Study the drawing (mm; zero at the part's minimum x, y, z) and answer. Give positions to 0.01 mm unless a question says otherwise; leave off trailing zeros. Write each loop counter-clockwise with the first axis right and the second up, starting at its lowest first coordinate (ties: lowest second). Pieces come first, ordered by that corner, then holes. Notation, with made-up numbers: (-12, 66) -> (14, 66) arc R29 ccw to (14, 90) -> close; hole circle Ø8 at (-33.5, 67). An arc over 180 degrees is marked (long way). One line per question, with ' | ' between items.
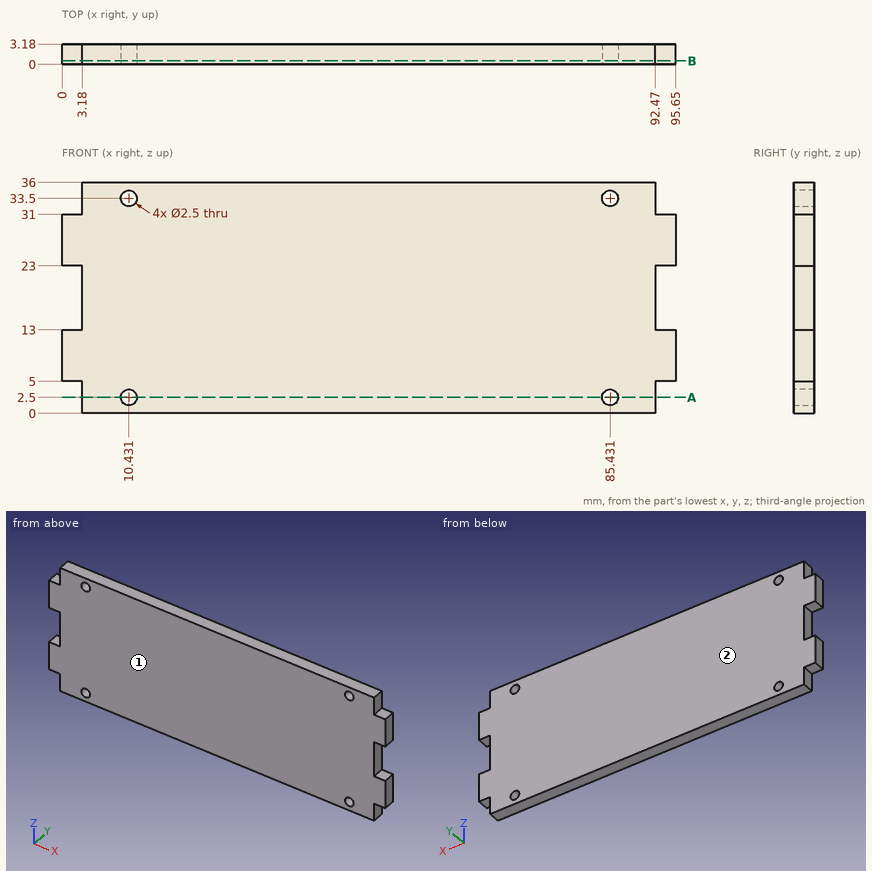
Item 1: Find section A-A (z = 2.5). Write down the section's boundary in (x, y).
Answers below:
outline: (3.18, 0) -> (9.18, 0) -> (9.18, 3.18) -> (3.18, 3.18) -> close; (11.68, 0) -> (84.18, 0) -> (84.18, 3.18) -> (11.68, 3.18) -> close; (86.68, 0) -> (92.47, 0) -> (92.47, 3.18) -> (86.68, 3.18) -> close
Item 2: Determine the mould class of the marked faces 1 and 2 for opening direction Y: pulls with the +Y half, pulls with the -Y half, needs draft (parallel to the pull), parting line crosses it, or undercut.
Answers below:
face 1: pulls with the -Y half | face 2: pulls with the +Y half
Item 3: Consider line 1 (X direction, y = 1.25, z = 33.5); line 2 (X direction, y = 1.8, z = 15); line 3 (Z direction, x = 9.5, y = 2.6) (1 decimal). Determine where each line is inside the solid, lowest interval first. Write a range as [from, to].
Answers below:
line 1: [3.18, 9.18], [11.68, 84.18], [86.68, 92.47] | line 2: [3.18, 92.47] | line 3: [0, 1.7], [3.3, 32.7], [34.3, 36]
Item 4: Find section B-B (y = 0.55). Write down the section's boundary in (x, z), then the cut area to 3 significant figures.
Answers below:
outline: (0, 5) -> (3.18, 5) -> (3.18, 0) -> (92.47, 0) -> (92.47, 5) -> (95.65, 5) -> (95.65, 13) -> (92.47, 13) -> (92.47, 23) -> (95.65, 23) -> (95.65, 31) -> (92.47, 31) -> (92.47, 36) -> (3.18, 36) -> (3.18, 31) -> (0, 31) -> (0, 23) -> (3.18, 23) -> (3.18, 13) -> (0, 13) -> close; hole circle Ø2.5 at (10.43, 2.5); hole circle Ø2.5 at (10.43, 33.5); hole circle Ø2.5 at (85.43, 2.5); hole circle Ø2.5 at (85.43, 33.5) | area: 3,300 mm²
Item 5: Flat-ended cylindrical pins translate along their axes: pin 1 (1.6 mm diameter, centred on x = 1.5, y = 1, fed in from -Z); pin 2 (1 mm diameter, centred on y = 2.5, z = 21.5, fed in from +X); pin 3 (1.6 mm diameter, centred on y = 1, z = 34, fed in from -X); pin 4 (2 mm diameter, centred on x = 85.43, z = 33.5, fed in from +Y). Find the tip coordinate at first contact, or state that the pin passes through.
Answers below:
pin 1: z = 5 | pin 2: x = 92.47 | pin 3: x = 3.18 | pin 4: through
